```python
from build123d import *

# Parameters (mm, degrees)
SKETCH2_W           = 34.5
SKETCH2_H           = 45
BOSS_EXTRUDE1_DEPTH = 3
SKETCH3_W           = 3
SKETCH3_H           = 45
BOSS_EXTRUDE2_DEPTH = 5.5
SKETCH4_W           = 22
SKETCH4_H           = 7
CUT_EXTRUDE1_DEPTH  = 8
FILLET1_R           = 3.5


with BuildPart() as part:
    # Sketch2 → Boss-Extrude1 (new body)
    with BuildSketch(Plane(origin=(0, 0, 0), x_dir=(1, 0, 0), z_dir=(0, 1, 0))):
        Rectangle(SKETCH2_W, SKETCH2_H)
    extrude(amount=BOSS_EXTRUDE1_DEPTH)

    # Sketch3 → Boss-Extrude2 (add)
    with BuildSketch(Plane(origin=(0, 3, 0), x_dir=(1, 0, 0), z_dir=(0, 1, 0))):
        with Locations((-15.75, 0)):
            Rectangle(SKETCH3_W, SKETCH3_H)
        with Locations((15.75, 0)):
            Rectangle(SKETCH3_W, SKETCH3_H)
    extrude(amount=BOSS_EXTRUDE2_DEPTH)

    # Sketch4 → Cut-Extrude1 (cut)
    with BuildSketch(Plane.XZ):
        with Locations((0, 13)):
            Rectangle(SKETCH4_W, SKETCH4_H)
        Rectangle(SKETCH4_W, SKETCH4_H)
        with Locations((0, -13)):
            Rectangle(SKETCH4_W, SKETCH4_H)
    extrude(amount=-CUT_EXTRUDE1_DEPTH, mode=Mode.SUBTRACT)

    # Fillet1
    fillet1_edges = [part.edges().sort_by_distance(p)[0] for p in [
        (-11, 1.5, -9.5),
        (-11, 1.5, -16.5),
        (11, 1.5, -9.5),
        (11, 1.5, -16.5),
        (11, 1.5, -3.5),
        (-11, 1.5, -3.5),
        (-11, 1.5, 3.5),
        (11, 1.5, 3.5),
        (11, 1.5, 9.5),
        (11, 1.5, 16.5),
        (-11, 1.5, 9.5),
        (-11, 1.5, 16.5),
    ]]
    fillet(fillet1_edges, radius=FILLET1_R - 0.0001)  # a hair under: the kernel refuses the full size


solid = part.part
```
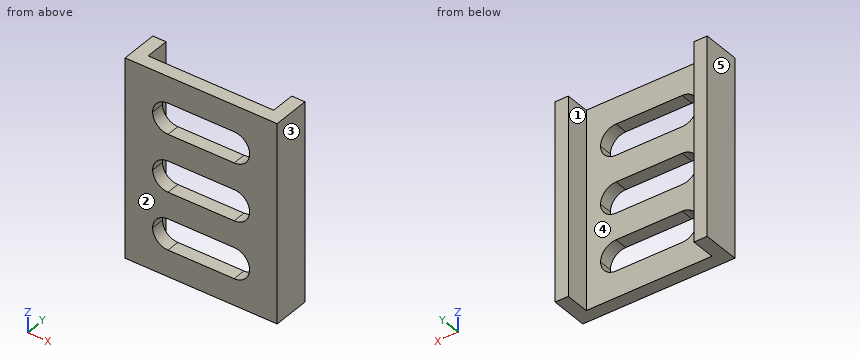
Can you work these out from the model? Positions are in its coordinate system, mm. Face numbers are marked on the shaded views. A direction names the side the tool comes from. Coordinates: 2 decimals unless noted, no trailing zeros. Order: outer loops, then holes, each group sorted by start corner. A loop starts at its lowest first (then second) coordinate and runs counter-clockwise, first axis right, second up. Notation, with made-up numbers: (71.25, -29) -> (105.25, -29) arc R14 ccw to (105.25, -6) -> close; hole circle Ø9 at (-12, 64). An arc over 180 degrees is marked (long way). Write each question's results on one line, items separated by ' | '.
Item 1: I want a section at B-B, the plane y = 6.5. Write out the boundary of the cut face in (x, z).
Results are:
outline: (-17.25, -22.5) -> (-14.25, -22.5) -> (-14.25, 22.5) -> (-17.25, 22.5) -> close; (14.25, -22.5) -> (17.25, -22.5) -> (17.25, 22.5) -> (14.25, 22.5) -> close
Item 2: I'm going to push a flat-ended pin straight in: pin 1 Ø1.5 at (x, z) = (7, -5.5) entering from +Y. Where does the tip first touch, or does it pass through?
Results are:
pin 1: y = 3
Item 3: If I drill on line 1 along Z through (x, y) = (6, 2); line 2 along X through (y, z) = (4.25, -20.5); line 3 along X through (y, z) = (0.75, 14), over which ranges is the centre line in solid material (lowest first)?
Results are:
line 1: -22.5 to -16.5, -9.5 to -3.5, 3.5 to 9.5, 16.5 to 22.5 | line 2: -17.25 to -14.25, 14.25 to 17.25 | line 3: -17.25 to -10.85, 10.85 to 17.25
Item 4: I want a section at A-A, the plane x = -2. Write out the boundary of the cut face in (y, z).
Results are:
outline: (0, -22.5) -> (3, -22.5) -> (3, -16.5) -> (0, -16.5) -> close; (0, -9.5) -> (3, -9.5) -> (3, -3.5) -> (0, -3.5) -> close; (0, 3.5) -> (3, 3.5) -> (3, 9.5) -> (0, 9.5) -> close; (0, 16.5) -> (3, 16.5) -> (3, 22.5) -> (0, 22.5) -> close
Item 5: Which directions (+Z, -Z, +X, -X, +Y, -Y) give clear straight access to the entire face, cutting with the end or side of a thin tool? Please do the marked faces 4 and 5.
Results are:
face 4: +Z, -Z, +Y | face 5: +Z, -Z, -X, +Y, -Y
Item 6: I want a section at C-C, the plane z = -8.5. Write out the boundary of the cut face in (x, y), then the cut area to 4 significant figures.
Results are:
outline: (-17.25, 0) -> (17.25, 0) -> (17.25, 8.5) -> (14.25, 8.5) -> (14.25, 3) -> (-14.25, 3) -> (-14.25, 8.5) -> (-17.25, 8.5) -> close | area: 136.5 mm²
Item 7: If we mould it in two halves opening along X, with no side actions, what happens to the marked faces 1, 2 and 3? For each: +X half, -X half, draft (parallel to the pull), parting line (faces both ways), or undercut.
Results are:
face 1: undercut | face 2: draft | face 3: +X half
Item 8: I want a section at D-D, the plane y = 2.25. Count the separate pieces of the cut face and the enclosed holes in it, then the cut area to 3 significant figures.
Results are:
separate pieces: 1 | enclosed holes: 3 | area: 1,120 mm²
